Part print with two shaded views. Sizes in mm from the minimum x, y, z corner. Give positions to 0.01 mm unless a question says otherwise; leave off trailing zeros. Order: outer loops, then holes, each group sorted by start corner. A loop starts at its lowest first (then second) coordinate and runs counter-clockwise, first axis right, second up. Notation, with made-up numbers: (70, 62) -> (113, 62) arc R30 ccw to (113, 92) -> close; hole circle Ø6 at (-31.5, 84.25). An arc over 180 degrees is marked (long way). Write item = value, one per line. Start each with the question number.
Item 1: Drill centre lines: line 1 along Y through (x, z) = (8.5, 0.3); line 2 along X through (y, z) = (9.5, 0.95); line 3 along Y through (x, z) = (16, 0.9). Where is each one in solid material? Low to high.
Item 2: Band-saw the part on C-C on y = 42. Write the cut outline in (x, z).
Item 3: Band-saw the part on B-B on z = 2.4. Count the separate pieces of the cut face and the enclosed holes in it, plus the area to 3 significant figures.
Item 4: Band-saw the part on D-D on x = 11. Write the cut outline in (y, z), plus the area to 3 significant figures.
Item 5: Flat gauge pins, fed straight in: P1, Ø0.9, axis at y = 1, z = 1.5, coming from the -X side; P2, Ø1.5, axis at x = 9.5, z = 2, coming from the +Y side; P3, Ø0.9, axis at y = 50.5, z = 1, coming from the +X side. Where does each tip first touch, or does it go through?
Item 6: Band-saw the part on A-A on y = 9.5. Write the cut outline in (x, z), plus the area to 3 significant figures.
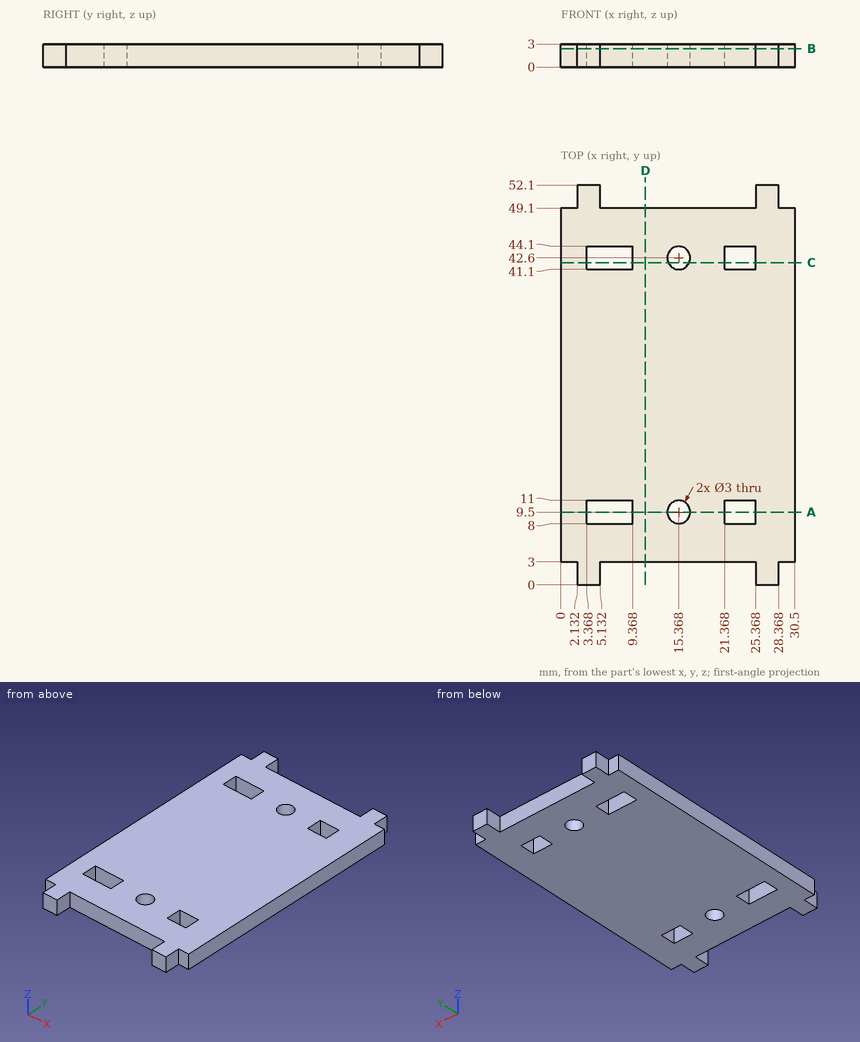
Values found:
q1.line_1 = 3 to 8, 11 to 41.1, 44.1 to 49.1
q1.line_2 = 0 to 3.37, 9.37 to 13.87, 16.87 to 21.37, 25.37 to 30.5
q1.line_3 = 3 to 8.14, 10.86 to 41.24, 43.96 to 49.1
q2.outline = (0, 0) -> (3.37, 0) -> (3.37, 3) -> (0, 3) -> close; (9.37, 0) -> (13.99, 0) -> (13.99, 3) -> (9.37, 3) -> close; (16.74, 0) -> (21.37, 0) -> (21.37, 3) -> (16.74, 3) -> close; (25.37, 0) -> (30.5, 0) -> (30.5, 3) -> (25.37, 3) -> close
q3.separate_pieces = 1
q3.enclosed_holes = 6
q3.area = 1,370 mm^2
q4.outline = (3, 0) -> (49.1, 0) -> (49.1, 3) -> (3, 3) -> close
q4.area = 138 mm^2
q5.P1 = 2.13
q5.P2 = 49.1
q5.P3 = 28.37
q6.outline = (0, 0) -> (3.37, 0) -> (3.37, 3) -> (0, 3) -> close; (9.37, 0) -> (13.87, 0) -> (13.87, 3) -> (9.37, 3) -> close; (16.87, 0) -> (21.37, 0) -> (21.37, 3) -> (16.87, 3) -> close; (25.37, 0) -> (30.5, 0) -> (30.5, 3) -> (25.37, 3) -> close
q6.area = 52.5 mm^2
